from build123d import *

# Parameters (mm, degrees)
SKETCH_1_W           = 15
SKETCH_1_H           = 15
EXTRUDE_1_DEPTH      = 15
SKETCH_2_W           = 11.5
SKETCH_2_H           = 13.5
CUT_EXTRUDE_1_DEPTH  = 11.5
CUT_EXTRUDE_2_DEPTH  = 9.45
SKETCH_4_W           = 3
SKETCH_4_H           = 3
EXTRUDE_2_DEPTH      = 1
EXTRUDE_3_DEPTH      = 2
EXTRUDE_3_DEPTH_BACK = 4
CUT_EXTRUDE_3_REACH  = 26.911
SKETCH_6_W           = 0.944409721
SKETCH_6_H           = 0.55
SKETCH_6_H_2         = 1.55
FILLET_1_R           = 0.1
FILLET_2_R           = 0.2


with BuildPart() as part:
    # 草图1 → 凸台-拉伸1 (new body)
    with BuildSketch(Plane.XY):
        with Locations((0, 7.5)):
            Rectangle(SKETCH_1_W, SKETCH_1_H)
    extrude(amount=-EXTRUDE_1_DEPTH)

    # 草图2 → 切除-拉伸1 (cut)
    with BuildSketch(Plane(origin=(0, 15, 0), x_dir=(-1, 0, 0), z_dir=(0, 1, 0))):
        with Locations((-1.75, -6.75)):
            Rectangle(SKETCH_2_W, SKETCH_2_H)
    extrude(amount=-CUT_EXTRUDE_1_DEPTH, mode=Mode.SUBTRACT)

    # 草图3 → 切除-拉伸2 (cut)
    with BuildSketch(Plane.XY):
        with BuildLine():
            Line((-1.5, 0), (-1.5, 0.677124344))
            ThreePointArc((-1.5, 0.677124344), (-1.780042303, 1.088161527), (-1.95, 1.555590279))
            Line((-1.95, 1.555590279), (-1.95, 2.8))
            Line((-1.95, 2.8), (1.95, 2.8))
            Line((1.95, 2.8), (1.95, 1.555590279))
            ThreePointArc((1.95, 1.555590279), (1.780042303, 1.088161527), (1.5, 0.677124344))
            Line((1.5, 0.677124344), (1.5, 0))
            Line((1.5, 0), (-1.5, 0))
        make_face()
        with BuildLine():
            Line((-7.5, 9), (-7.5, 6))
            Line((-7.5, 6), (-6.822875656, 6))
            ThreePointArc((-6.822875656, 6), (-6.411838473, 5.719957697), (-5.944409721, 5.55))
            Line((-5.944409721, 5.55), (-4.7, 5.55))
            Line((-4.7, 5.55), (-4.7, 9.45))
            Line((-4.7, 9.45), (-5.944409721, 9.45))
            ThreePointArc((-5.944409721, 9.45), (-6.411838473, 9.280042303), (-6.822875656, 9))
            Line((-6.822875656, 9), (-7.5, 9))
        make_face()
    extrude(amount=-CUT_EXTRUDE_2_DEPTH, mode=Mode.SUBTRACT)

    # 草图4 → 凸台-拉伸2 (add)
    with BuildSketch(Plane(origin=(0, 0, -15), x_dir=(-1, 0, 0), z_dir=(0, 0, -1))):
        with Locations((0, 7.5)):
            Rectangle(SKETCH_4_W, SKETCH_4_H)
    extrude(amount=EXTRUDE_2_DEPTH)

    # 草图5 → 凸台-拉伸3 (add, two sides: drawn at the far end of the back side and taken through both)
    with BuildSketch(Plane(origin=(0, 9, 0), x_dir=(-1, 0, 0), z_dir=(0, 1, 0)).offset(-EXTRUDE_3_DEPTH_BACK)):
        with BuildLine():
            Line((1.95, -17.5), (-1.95, -17.5))
            Line((-1.95, -17.5), (-1.95, -16.555590279))
            ThreePointArc((-1.95, -16.555590279), (-1.780042303, -16.088161527), (-1.5, -15.677124344))
            Line((-1.5, -15.677124344), (1.5, -15.677124344))
            ThreePointArc((1.5, -15.677124344), (1.780042303, -16.088161527), (1.95, -16.555590279))
            Line((1.95, -16.555590279), (1.95, -17.5))
        make_face()
    extrude(amount=EXTRUDE_3_DEPTH + EXTRUDE_3_DEPTH_BACK)

    # 草图6 → 切除-拉伸3 (cut, up to next)
    with BuildSketch(Plane(origin=(1.95, 0, 0), x_dir=(0, 0, -1), z_dir=(1, 0, 0)), mode=Mode.PRIVATE) as cut_extrude_3_sk1:
        with BuildLine():
            Line((16.555590279, 5), (16.555590279, 5.55))
            ThreePointArc((16.555590279, 5.55), (16.088161527, 5.719957697), (15.677124344, 6))
            Line((15.677124344, 6), (15.677124344, 5))
            Line((15.677124344, 5), (16.555590279, 5))
        make_face()
    cut_extrude_3_tool1 = extrude(cut_extrude_3_sk1.sketch, amount=-CUT_EXTRUDE_3_REACH, mode=Mode.PRIVATE) & part.part
    # 草图6 → 切除-拉伸3 (cut, up to next)
    with BuildSketch(Plane(origin=(1.95, 0, 0), x_dir=(0, 0, -1), z_dir=(1, 0, 0)), mode=Mode.PRIVATE) as cut_extrude_3_sk2:
        with Locations((17.02779514, 5.275)):
            Rectangle(SKETCH_6_W, SKETCH_6_H)
    cut_extrude_3_tool2 = extrude(cut_extrude_3_sk2.sketch, amount=-CUT_EXTRUDE_3_REACH, mode=Mode.PRIVATE) & part.part
    # 草图6 → 切除-拉伸3 (cut, up to next)
    with BuildSketch(Plane(origin=(1.95, 0, 0), x_dir=(0, 0, -1), z_dir=(1, 0, 0)), mode=Mode.PRIVATE) as cut_extrude_3_sk3:
        with Locations((17.02779514, 10.225)):
            Rectangle(SKETCH_6_W, SKETCH_6_H_2)
    cut_extrude_3_tool3 = extrude(cut_extrude_3_sk3.sketch, amount=-CUT_EXTRUDE_3_REACH, mode=Mode.PRIVATE) & part.part
    # 草图6 → 切除-拉伸3 (cut, up to next)
    with BuildSketch(Plane(origin=(1.95, 0, 0), x_dir=(0, 0, -1), z_dir=(1, 0, 0)), mode=Mode.PRIVATE) as cut_extrude_3_sk4:
        with BuildLine():
            ThreePointArc((15.677124344, 9), (16.088161527, 9.280042303), (16.555590279, 9.45))
            Line((16.555590279, 9.45), (16.555590279, 11))
            Line((16.555590279, 11), (15.677124344, 11))
            Line((15.677124344, 11), (15.677124344, 9))
        make_face()
    cut_extrude_3_tool4 = extrude(cut_extrude_3_sk4.sketch, amount=-CUT_EXTRUDE_3_REACH, mode=Mode.PRIVATE) & part.part
    add(cut_extrude_3_tool1.solids().sort_by_distance((1.95, 5.375771, -16.07186))[0], mode=Mode.SUBTRACT)
    add(cut_extrude_3_tool2.solids().sort_by_distance((1.95, 5.275, -17.027795))[0], mode=Mode.SUBTRACT)
    add(cut_extrude_3_tool3.solids().sort_by_distance((1.95, 10.225, -17.027795))[0], mode=Mode.SUBTRACT)
    add(cut_extrude_3_tool4.solids().sort_by_distance((1.95, 10.130885, -16.097603))[0], mode=Mode.SUBTRACT)

    # 圆角1
    fillet_1_edges = [part.edges().sort_by_distance(p)[0] for p in [
        (1.95, 7.5, -17.5),
        (-1.95, 7.5, -17.5),
        (0, 5.55, -17.5),
        (0, 9.45, -17.5),
    ]]
    fillet(fillet_1_edges, radius=FILLET_1_R)

    # 圆角2
    fillet_2_edges = [part.edges().sort_by_distance(p)[0] for p in [
        (7.5, 7.5, -15),
        (0, 15, -15),
        (-5.75, 15, 0),
        (4.5, 0, 0),
        (0, 0, -9.45),
        (1.5, 0, -4.725),
        (-1.5, 0, -4.725),
        (-7.5, 7.5, -15),
        (7.5, 1.75, 0),
        (-7.5, 3, 0),
        (-4.5, 0, 0),
        (-7.5, 7.5, -9.45),
        (-7.5, 6, -4.725),
        (-7.5, 9, -4.725),
        (-7.5, 12, 0),
        (0, 0, -15),
        (-7.5, 15, -7.5),
        (7.5, 15, -14.25),
        (7.5, 0, -7.5),
        (-7.5, 0, -7.5),
    ]]
    fillet(fillet_2_edges, radius=FILLET_2_R)


solid = part.part
Could you check a few things on this model? Use its own coordinates, in mm. A direction names the side the tool comes from. Round coordinates to 2 decimals unless told otherwise and drop trailing zeros. Write each loop counter-clockwise with the first axis right and the second up, starting at its lowest first coordinate (ties: lowest second). Pieces come first, ordered by that corner, then holes. Notation, with made-up numbers: (63.25, -35) - (107.25, -35) arc R20 cw to (107.25, -21) - close; hole circle Ø3 at (-18.75, -34.75). An arc over 180 degrees is marked (long way). Use a Markdown table: item, result.
Q1. I want a section at C-C (y = 7.75). List the corners of the cut face in (x, z) for me, plus the area to 3 significant figures.
Output values:
| item | result |
|---|---|
| outline | (-7.5, -14.8) arc R0.2 ccw to (-7.3, -15) - (-1.5, -15) - (-1.5, -15.68) arc R2 ccw to (-1.95, -16.56) - (-1.95, -17.4) arc R0.1 ccw to (-1.85, -17.5) - (1.85, -17.5) arc R0.1 ccw to (1.95, -17.4) - (1.95, -16.56) arc R2 ccw to (1.5, -15.68) - (1.5, -15) - (7.3, -15) arc R0.2 ccw to (7.5, -14.8) - (7.5, -13.5) - (-4, -13.5) - (-4, 0) - (-4.7, 0) - (-4.7, -9.45) - (-7.3, -9.45) arc R0.2 ccw to (-7.5, -9.65) - close |
| area | 52.1 mm2 |
Q2. Please list where these lines run through material, in increasing order: L1, parallel to X at y = 2.5, z = -3.5; L2, parallel to Y at x = 3.5, z = -5.75; L3, parallel to X at y = 7, z = -15.25.
Output values:
| item | result |
|---|---|
| L1 | -7.5 to -1.95, 1.95 to 7.5 |
| L2 | 0 to 3.5 |
| L3 | -1.5 to 1.5 |
Q3. I want a section at D-D (x = 4.75). List the corners of the cut face in (y, z) for me.
Output values:
| item | result |
|---|---|
| outline | (0, -14.8) arc R0.2 ccw to (0.2, -15) - (14.8, -15) arc R0.2 ccw to (15, -14.8) - (15, -13.5) - (3.5, -13.5) - (3.5, 0) - (0.2, 0) arc R0.2 ccw to (0, -0.2) - close |
Q4. I want a section at B-B (z = -11). List the corners of the cut face in (x, y) for me.
Output values:
| item | result |
|---|---|
| outline | (-7.5, 0.2) arc R0.2 ccw to (-7.3, 0) - (7.3, 0) arc R0.2 ccw to (7.5, 0.2) - (7.5, 3.5) - (-4, 3.5) - (-4, 15) - (-7.3, 15) arc R0.2 ccw to (-7.5, 14.8) - close |
Q5. For faces 4 (the flat face through (1.95, 7, -17)), 5 (the cylindrical face through (-1.777, 7.473, -16.082)), 6 (the cylindrical face through (0.027, 9.277, -16.082)), 7 (the flat face through (-6, 8, -9.45)), which set-ups out of +Z, -Z, +X, -X, +Y, -Y let a thin tool reach every point of the face, with its end or its side?
Output values:
| item | result |
|---|---|
| face 4 | -Z, +X, +Y, -Y |
| face 5 | -X, +Y, -Y |
| face 6 | +X, -X, +Y |
| face 7 | +Z |
Q6. For pin 1 (1 mm diameter, centred on x = -4.5, y = 7, fed in from +Z); pin 2 (0.8 mm diameter, centred on x = 0.5, y = 1, fed in from +Z); pin 3 (1 mm diameter, centred on y = 4.5, z = -11.5, fed in from +X); pin 4 (0.7 mm diameter, centred on y = 7, z = -17, fed in from +X), each with a flat end and sliding along its axis, tell me the tip position at first contact or that it passes through.
Output values:
| item | result |
|---|---|
| pin 1 | z = 0 |
| pin 2 | z = -9.45 |
| pin 3 | x = -4 |
| pin 4 | x = 1.95 |
Q7. Thinking about a two-plate mould opening in X: for faces 1 (the flat face through (0, 2.8, -5)), 2 (the flat face through (-7.5, 7, -11)), 3 (the flat face through (-4.4, 15, -9.1)), which applies, released by +X, released by -X, zero draft, split by the parting line, or undercut?
Output values:
| item | result |
|---|---|
| face 1 | undercut |
| face 2 | released by -X |
| face 3 | zero draft |
Q8. I want a section at A-A (x = 0.75). List the corners of the cut face in (y, z) for me, plus the area to 3 significant figures.
Output values:
| item | result |
|---|---|
| outline | (0, -14.8) arc R0.2 ccw to (0.2, -15) - (6, -15) - (6, -15.68) arc R2 ccw to (5.55, -16.56) - (5.55, -17.4) arc R0.1 ccw to (5.65, -17.5) - (9.35, -17.5) arc R0.1 ccw to (9.45, -17.4) - (9.45, -16.56) arc R2 ccw to (9, -15.68) - (9, -15) - (14.8, -15) arc R0.2 ccw to (15, -14.8) - (15, -13.5) - (3.5, -13.5) - (3.5, 0) - (2.8, 0) - (2.8, -9.45) - (0.2, -9.45) arc R0.2 ccw to (0, -9.65) - close |
| area | 52.1 mm2 |
